Verification items for the finished model (mm, model axes). Face numbers are marked on the shaded views. A direction names the side the tool comes from. Give positions to 0.01 mm unless a question says otherwise; leave off trailing zeros. Order: outer loops, then holes, each group sorted by start corner. A loop starts at its lowest first (then second) coordinate and runs counter-clockwise, first axis right, second up. Notation, with made-up numbers: (10, -23) -> (32, -23) arc R23 ccw to (32, -14) -> close; hole circle Ø1 at (13, -24.75). An arc over 180 degrees is marked (long way). Return JSON: item names as keys, results as strings. Group by question number.
(1) Cross-section at C-C on x = 14.5. Enter the section's corners in (y, z), then the cut area to 3 significant figures.
(2) Depth check by flat-ended pin: pin 1 Ø1.5 at (y, z) = (1.5, 4) entering from +X; pin 2 Ø4.5 at (x, y) = (45.5, -0.5) entering from +Z; pin 3 Ø3 at (x, z) = (37, 4) entering from -Y. Enter the tip coordinate at first touch or a pass-through.
(3) Cross-section at B-B on y = -1.5. Enter the section's corners in (x, z), then the cut area to 3 significant figures.
(4) Tool access check on the marked faces 1 and 2. Record the directions out of +Z, -Z, +X, -X, +Y, -Y that give a thin tool (end or side, any length) a straight path to the whole face; none if there is none.
(5) Thickness scan on line 1 along X through (y, z) = (-0.5, 2.05); line 2 along X through (y, z) = (1.5, 0.6); line 3 along Y through (x, z) = (14.5, 1.3). Record the ranges inside material, lowest first.
(6) Cross-section at D-D on z = 2.25. Enter the section's corners in (x, y), then the cut area to 3 significant figures.
(7) Cross-section at A-A on z = 4.05. Enter the section's corners in (x, y).
from build123d import *

# Parameters (mm, degrees)
BOSS_EXTRUDE1_DEPTH     = 5
CUT_EXTRUDE1_DEPTH      = 53.75142939
CUT_EXTRUDE1_DEPTH_BACK = 53.75142939
SKETCH2_R               = 1.75
SKETCH5_R               = 3
CUT_EXTRUDE2_DEPTH      = 2


with BuildPart() as part:
    # Sketch1 → Boss-Extrude1 (new body)
    with BuildSketch(Plane.XY):
        with BuildLine():
            Line((23.11684397, 8), (36.88315603, 8))
            Line((36.88315603, 8), (46.90520921, 5.744848006))
            ThreePointArc((46.90520921, 5.744848006), (51.591551748, -2.466147717), (42.989140572, -6.387981358))
            Line((42.989140572, -6.387981358), (34.244441462, -2.658908715))
            ThreePointArc((34.244441462, -2.658908715), (30, -2), (25.755558538, -2.658908715))
            Line((25.755558538, -2.658908715), (17.05409045, -6.415729603))
            ThreePointArc((17.05409045, -6.415729603), (8.36828995, -2.480244081), (13.111532947, 5.792169261))
            Line((13.111532947, 5.792169261), (23.11684397, 8))
        make_face()
    extrude(amount=BOSS_EXTRUDE1_DEPTH)

    # Sketch2 → Cut-Extrude1 (cut, two sides: drawn at the far end of the back side and taken through both)
    with BuildSketch(Plane.XY.offset(5).offset(-CUT_EXTRUDE1_DEPTH_BACK)):
        with Locations((45.5, -0.5)):
            Circle(SKETCH2_R)
        with Locations((14.5, -0.5)):
            Circle(SKETCH2_R)
        with Locations((26, 3)):
            Circle(SKETCH2_R)
        with Locations((34, 3)):
            Circle(SKETCH2_R)
    extrude(amount=CUT_EXTRUDE1_DEPTH + CUT_EXTRUDE1_DEPTH_BACK, mode=Mode.SUBTRACT)

    # Sketch5 → Cut-Extrude2 (cut)
    with BuildSketch(Plane.XY.offset(5)):
        with Locations((26, 3)):
            Circle(SKETCH5_R)
        with Locations((34, 3)):
            Circle(SKETCH5_R)
        with Locations((45.5, -0.5)):
            Circle(SKETCH5_R)
        with Locations((14.5, -0.5)):
            Circle(SKETCH5_R)
    extrude(amount=-CUT_EXTRUDE2_DEPTH, mode=Mode.SUBTRACT)


solid = part.part
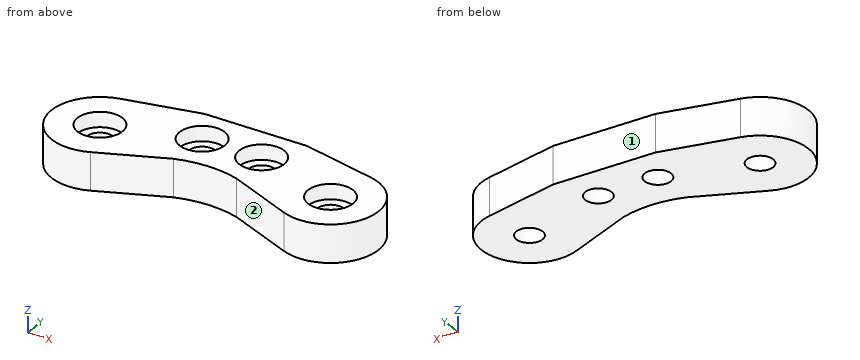
Verdict:
{
 "1": {"outline": "(-6.94, 0) -> (-2.25, 0) -> (-2.25, 3) -> (-3.5, 3) -> (-3.5, 5) -> (-6.94, 5) -> close; (1.25, 0) -> (6.1, 0) -> (6.1, 5) -> (2.5, 5) -> (2.5, 3) -> (1.25, 3) -> close", "area": "42.7 mm²"},
 "2": {"pin 1": "x = 51.78", "pin 2": "z = 3", "pin 3": "y = -4.47"},
 "3": {"outline": "(8.13, 0) -> (13.06, 0) -> (13.06, 3) -> (11.67, 3) -> (11.67, 5) -> (8.13, 5) -> close; (15.94, 0) -> (44.06, 0) -> (44.06, 3) -> (42.67, 3) -> (42.67, 5) -> (17.33, 5) -> (17.33, 3) -> (15.94, 3) -> close; (46.94, 0) -> (51.82, 0) -> (51.82, 5) -> (48.33, 5) -> (48.33, 3) -> (46.94, 3) -> close", "area": "179 mm²"},
 "4": {"face 1": "+Z, -Z, +X, -X, +Y", "face 2": "+Z, -Z, -Y"},
 "5": {"line 1": "8.06 to 12.75, 16.25 to 43.75, 47.25 to 51.9", "line 2": "8.37 to 25.1, 26.9 to 33.1, 34.9 to 51.58", "line 3": "-6.94 to -2.25, 1.25 to 6.1"},
 "6": {"outline": "(13.11, 5.79) arc R6.44 ccw (long way) to (17.05, -6.42) -> (25.76, -2.66) arc R14 cw to (34.24, -2.66) -> (42.99, -6.39) arc R6.4 ccw (long way) to (46.91, 5.74) -> (36.88, 8) -> (23.12, 8) -> close; hole circle Ø3.5 at (14.5, -0.5); hole circle Ø3.5 at (26, 3); hole circle Ø3.5 at (34, 3); hole circle Ø3.5 at (45.5, -0.5)", "area": "455 mm²"},
 "7": {"outline": "(13.11, 5.79) arc R6.44 ccw (long way) to (17.05, -6.42) -> (25.76, -2.66) arc R14 cw to (34.24, -2.66) -> (42.99, -6.39) arc R6.4 ccw (long way) to (46.91, 5.74) -> (36.88, 8) -> (23.12, 8) -> close; hole circle Ø6 at (14.5, -0.5); hole circle Ø6 at (26, 3); hole circle Ø6 at (34, 3); hole circle Ø6 at (45.5, -0.5)"}
}
